Read the model definition and answer for the solid it produces. Units are mm, in the model's axes. A direction names the side the tool comes from. Round coordinates to 2 decimals unless told otherwise and drop trailing zeros. Write each loop counter-clockwise with the first axis right and the second up, starting at its lowest first coordinate (ties: lowest second). Pieces come first, ordered by that corner, then holes. Notation, with made-up numbers: (73.5, -23) - (96.5, -23) arc R13 ccw to (96.5, -2) - close; hole circle Ø3 at (54.25, 79.25). An arc over 180 degrees is marked (long way). Use one line per item in the form item = value. Start each with the question number.
1) This flat-tipped pin is pushed along its axis until it touches: pin 1 (1.5 mm diameter, centred on x = 38.5, z = 3, fed in from -Y). Where does it stop, or does it pass through?
2) The part is cut by section A-A, the plane z = 2.35. Give the vertices of the cut face in (x, y), plus the area to 3 significant figures.
3) For faces 1 (the face through (-49, 30, 2)), 2 (the face through (-102, 15, 2)), 3 (the face through (76, 28, 2)), determine the directions among +Z, -Z, +X, -X, +Y, -Y from which every point of the face is accessible in a straight line to the end or side of a thin tool.
4) Consider line 1 along Y through (x, z) = (75, 2.1); line 2 along Y through (x, z) = (-70, 2.75); line 3 along Z through (x, y) = (-39, 31.5). Determine where each line is inside the solid, lowest interval first. Write a range as from..to.
from build123d import *

# Parameters (mm, degrees)
F1_DEPTH = 4
F2_SIZE  = 3.99999
F3_SIZE  = 3.99999
F4_SIZE  = 3.99999


# Not quite as in the source:
# - a fillet or chamfer is up to 0.001 mm smaller than in the source, because OpenCascade refuses the exact size


with BuildPart() as f1:
    # F0 (on Top) → F1 (new body)
    with BuildSketch(Plane.XY):
        Polygon((-102, 0), (0, 0), (102, 0), (102, 30), (49, 30), (49, 34), (-49, 34), (-49, 30), (-102, 30), align=None)
    extrude(amount=F1_DEPTH)

    # F2 (size 4 in the source; OpenCascade refuses exactly that, so slightly less here)
    f2_edges = [f1.edges().sort_by_distance(p)[0] for p in [
        (75.5, 30, 0),
    ]]
    chamfer(f2_edges, length=F2_SIZE)

    # F3 (size 4 in the source; OpenCascade refuses exactly that, so slightly less here)
    f3_edges = [f1.edges().sort_by_distance(p)[0] for p in [
        (0, 34, 0),
    ]]
    chamfer(f3_edges, length=F3_SIZE)

    # F4 (size 4 in the source; OpenCascade refuses exactly that, so slightly less here)
    f4_edges = [f1.edges().sort_by_distance(p)[0] for p in [
        (-75.5, 30, 0),
    ]]
    chamfer(f4_edges, length=F4_SIZE)


solid = f1.part
Geometry results:
q1.pin_1 = 0
q2.outline = (-102, 0) - (102, 0) - (102, 28.35) - (49, 28.35) - (49, 32.35) - (-49, 32.35) - (-49, 28.35) - (-102, 28.35) - close
q2.area = 6,180 mm2
q3.face_1 = -Z, -X, +Y
q3.face_2 = +Z, -Z, -X, +Y, -Y
q3.face_3 = -Z, +X, +Y
q4.line_1 = 0..28.1
q4.line_2 = 0..28.75
q4.line_3 = 1.5..4
